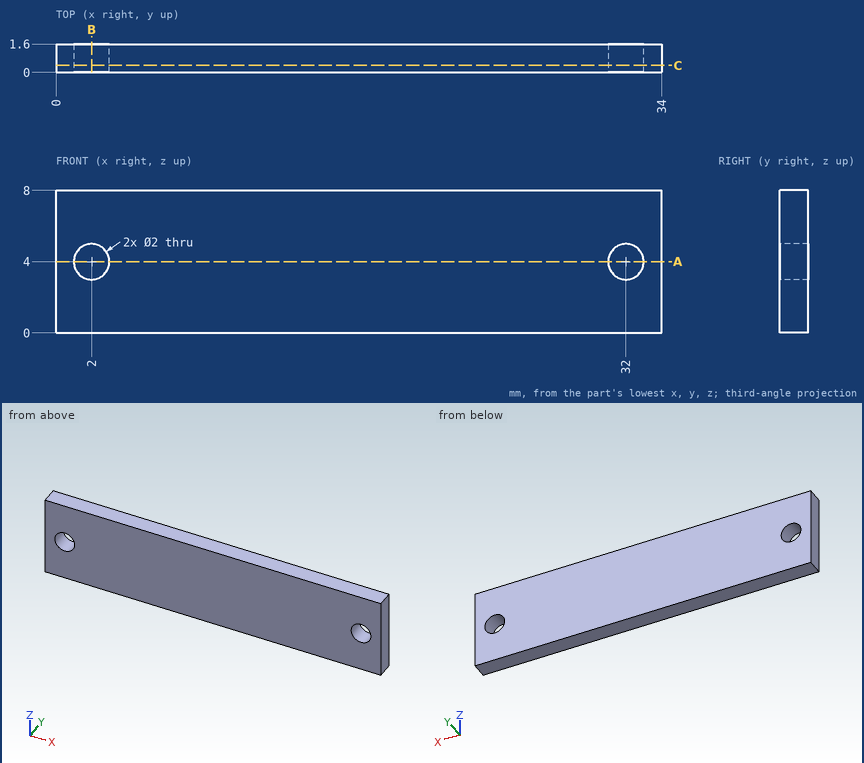
For this review, use the dimensioned drawing (mm, ordinates from the lowest corner) and the shaded views. Give positions to 0.01 mm unless a question says otherwise; leave off trailing zeros. Write each loop counter-clockwise with the first axis right and the second up, starting at its lowest first coordinate (ties: lowest second). Pieces come first, ordered by that corner, then holes. Notation, with made-up numbers: M 85,-23.75 L 134,-23.75 A31 ccw 134,1.25 Z; hole C 64.5,26.5 d4. An arc over 180 degrees is marked long. Answer as a JSON object with one key per item and string values. Group by question number.
Item 1: Consider section C-C on y = 0.4. Write out the cut boundary in (x, z).
Item 2: For pin 1 Ø1.6 at (x, z) = (2, 4) entering from +Y; pin 2 Ø2 at (x, z) = (14.5, 1.5) entering from -Y, all flat-tipped, find the tip position at first contact; note any pin that passes through.
Item 3: Consider section B-B on x = 2. Write out the cut boundary in (y, z), plus the area to 3 significant figures.
Item 4: Consider section A-A on z = 4. Write out the cut boundary in (x, y).
Item 5: For probe 1 along Z at (x, y) = (32, 0.4); probe 2 along X at (y, z) = (0.45, 4.5); probe 3 along Z at (x, y) = (32.5, 1.05), list the stretches that pass through material, from the lowest coordinate up. Write a range as [from, to].
Check result:
{
 "1": {"outline": "M 0,0 L 34,0 L 34,8 L 0,8 Z; hole C 2,4 d2; hole C 32,4 d2"},
 "2": {"pin 1": "passes through", "pin 2": "stops at y = 0"},
 "3": {"outline": "M 0,0 L 1.6,0 L 1.6,3 L 0,3 Z; M 0,5 L 1.6,5 L 1.6,8 L 0,8 Z", "area": "9.60 mm^2"},
 "4": {"outline": "M 0,0 L 1,0 L 1,1.6 L 0,1.6 Z; M 3,0 L 31,0 L 31,1.6 L 3,1.6 Z; M 33,0 L 34,0 L 34,1.6 L 33,1.6 Z"},
 "5": {"probe 1": "z = [0, 3], [5, 8]", "probe 2": "x = [0, 1.13], [2.87, 31.13], [32.87, 34]", "probe 3": "z = [0, 3.13], [4.87, 8]"}
}
